Could you check a few things on this model? Use its own coordinates, in mm. Face numbers are marked on the shaded views. A direction names the side the tool comes from. Coordinates: 2 decimals unless noted, no trailing zeros. Loops run counter-clockwise (first coordinate to the right, second up) from the corner with the lowest first, then second, coordinate; pieces in that order, holes last.
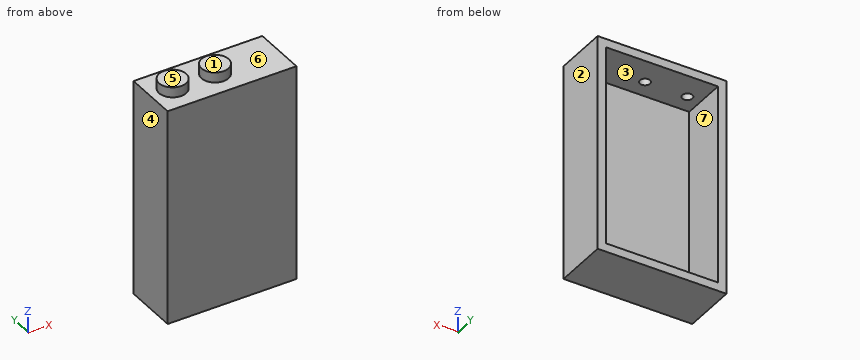
from build123d import *

# Parameters (mm, degrees)
SKETCH1_W           = 38
SKETCH1_H           = 64
BOSS_EXTRUDE1_DEPTH = 16
SKETCH2_R           = 4
BOSS_EXTRUDE2_DEPTH = 3
SHELL1_T            = -2.5


with BuildPart() as part:
    # Sketch1 → Boss-Extrude1 (new body)
    with BuildSketch(Plane(origin=(0, 0, 0), x_dir=(1, 0, 0), z_dir=(0, 1, 0))):
        with Locations((19, -32)):
            Rectangle(SKETCH1_W, SKETCH1_H)
    extrude(amount=BOSS_EXTRUDE1_DEPTH)

    # Sketch2 → Boss-Extrude2 (add)
    with BuildSketch(Plane.XY.offset(64)):
        with Locations((19, 8)):
            Circle(SKETCH2_R)
        with Locations((6.5, 8)):
            Circle(SKETCH2_R)
    extrude(amount=BOSS_EXTRUDE2_DEPTH)

    # Shell1
    shell1_openings = [part.faces().sort_by_distance(p)[0] for p in [
        (19, 16, 32),
    ]]
    offset(amount=SHELL1_T, openings=shell1_openings, kind=Kind.INTERSECTION)


solid = part.part
(1) Which directions (+Z, -Z, +X, -X, +Y, -Y) give clear straight access to the entire face, cutting with the end or side of a thin tool? Please do the marked faces 5, 6 and 7.
Answers:
face 5: +Z, +X, -X, +Y, -Y
face 6: +Z
face 7: +Y
(2) Imagine slicing it at B-B, the plane x = 26.5. Write out the boundary of the cut face in (y, z), and give its area (4 significant figures).
Answers:
outline: (0, 0) - (16, 0) - (16, 2.5) - (2.5, 2.5) - (2.5, 61.5) - (16, 61.5) - (16, 64) - (0, 64) - close
area: 227.5 mm2
(3) We'd pull the mould along X, two halves only. Please class the marked faces 1, 2, 3 and 4: +X half, -X half, draft (parallel to the pull), parting line (faces both ways), or undercut.
Answers:
face 1: draft
face 2: +X half
face 3: undercut
face 4: -X half
(4) For pin 1 (2 mm diameter, centred on x = 33.5, y = 8, fed in from +Z); pin 2 (2 mm diameter, centred on x = 24, z = 28, fed in from +Y), each with a flat end and sliding along its axis, tell me the tip position at first contact or that it passes through.
Answers:
pin 1: stops at z = 64
pin 2: stops at y = 2.5
(5) Imagine slicing it at C-C, the plane z = 8. Write out the boundary of the cut face in (x, y), and give its area (4 significant figures).
Answers:
outline: (0, 0) - (38, 0) - (38, 16) - (35.5, 16) - (35.5, 2.5) - (2.5, 2.5) - (2.5, 16) - (0, 16) - close
area: 162.5 mm2
(6) Imagine slicing it at A-A, the plane y = 8. Write out the boundary of the cut face in (x, z), and give its area (3 significant figures).
Answers:
outline: (0, 0) - (38, 0) - (38, 64) - (23, 64) - (23, 67) - (15, 67) - (15, 64) - (10.5, 64) - (10.5, 67) - (2.5, 67) - (2.5, 64) - (0, 64) - close; hole (2.5, 2.5) - (35.5, 2.5) - (35.5, 61.5) - (20.5, 61.5) - (20.5, 64.5) - (17.5, 64.5) - (17.5, 61.5) - (8, 61.5) - (8, 64.5) - (5, 64.5) - (5, 61.5) - (2.5, 61.5) - close
area: 515 mm2
(7) I need wall thicknesses on probe 1 along X at (y, z) = (8, 62.7); probe 2 along Z at (x, y) = (31, 12); probe 3 along Y at (x, z) = (19, 63.45). Which ranges of each line are inside material? Lowest first, please.
Answers:
probe 1: x = 0 to 5, 8 to 17.5, 20.5 to 38
probe 2: z = 0 to 2.5, 61.5 to 64
probe 3: y = 0 to 6.5, 9.5 to 16
(8) Imagine slicing it at D-D, the plane y = 14.75. Write out the boundary of the cut face in (x, z).
Answers:
outline: (0, 0) - (38, 0) - (38, 64) - (0, 64) - close; hole (2.5, 2.5) - (35.5, 2.5) - (35.5, 61.5) - (2.5, 61.5) - close
